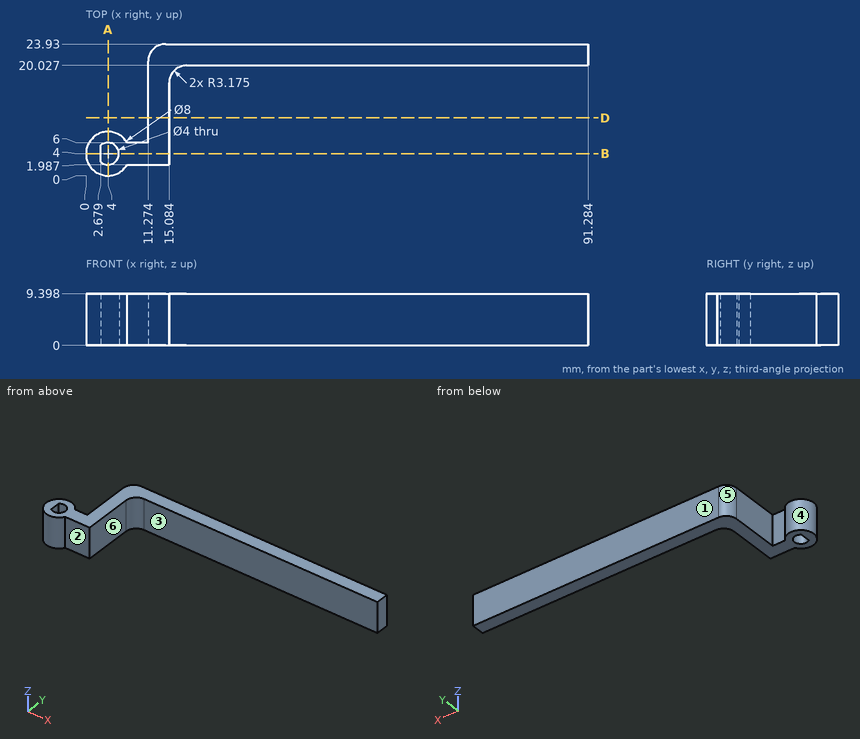
Job drawing, mm, ordinate dimensions from the low corner. One solid piece. A direction names the side the tool comes from. Round coordinates to 2 decimals unless told otherwise and drop trailing zeros. Order: outer loops, then holes, each group sorted by start corner. A loop starts at its lowest first (then second) coordinate and runs counter-clockwise, first axis right, second up. Notation, with made-up numbers: (30, -14.5) -> (49, -14.5) arc R25 cw to (49, 20.5) -> close; hole circle Ø8 at (63, -9.5). An arc over 180 degrees is marked (long way). Write item = value, one per line.
(1) Drill centre lines: L1, parallel to X at y = 4, z = 5.5; L2, parallel to Y at x = 4, z = 6; L3, parallel to Y at x = 87, z = 9.25. Where is each one in solid material? Low to high.
Answers follow:
L1 = 0 to 2.68, 6 to 15.08
L2 = 0 to 2, 6 to 8
L3 = 20.03 to 23.93
(2) Cut at A-A (x = 4). Write the cut outline in (y, z).
Answers follow:
outline = (0, 0) -> (2, 0) -> (2, 9.4) -> (0, 9.4) -> close; (6, 0) -> (8, 0) -> (8, 9.4) -> (6, 9.4) -> close
(3) Pull direction X, two halves, no side cores. Call the marked faces 3, 4, 5 and 6: +X half, -X half, draft (parallel to the pull), parting line (faces both ways), or undercut.
Answers follow:
face_3 = draft
face_4 = undercut
face_5 = -X half
face_6 = +X half
(4) 3-axis set-ups, long thin cutter, end or side, ignore diameter. For the marked faces 1 and 2: which of +Z, -Z, +X, -X, +Y, -Y reach the whole face in a straight line?
Answers follow:
face_1 = +Z, -Z, +X, -X, +Y
face_2 = +Z, -Z, +X, -Y
(5) Cut at D-D (y = 10.5). Write the cut outline in (x, z).
Answers follow:
outline = (11.27, 0) -> (15.08, 0) -> (15.08, 9.4) -> (11.27, 9.4) -> close
(6) Flat gauge pins, fed straight in: P1, Ø1.5, axis at x = 75, z = 2.5, coming from the -Y side; P2, Ø2.5, axis at y = 3.5, z = 5.5, coming from the +X side; P3, Ø2, axis at y = 17.5, z = 7, coming from the +X side (1 decimal); P4, Ø3.5, axis at x = 4, y = 4, coming from the -Z side. Where does each tip first touch, or does it go through?
Answers follow:
P1 = 20.03
P2 = 15.08
P3 = 15.5
P4 = 0
(7) Cut at B-B (y = 4). Write the cut outline in (x, z), plus the area to 3 significant figures.
Answers follow:
outline = (0, 0) -> (2.68, 0) -> (2.68, 9.4) -> (0, 9.4) -> close; (6, 0) -> (15.08, 0) -> (15.08, 9.4) -> (6, 9.4) -> close
area = 111 mm²
